```python
from build123d import *

# Parameters (mm, degrees)
SKETCH_1_R               = 9
SKETCH_1_R_2             = 6.25
EXTRUDE_1_DEPTH          = 200
SKETCH_2_R               = 1.75
CUT_EXTRUDE_1_DEPTH      = 10
CUT_EXTRUDE_1_DEPTH_BACK = 10


with BuildPart() as part:
    # ｽｹｯﾁ1 → ﾎﾞｽ - 押し出し1 (new body)
    with BuildSketch(Plane.XY):
        Circle(SKETCH_1_R)
        Circle(SKETCH_1_R_2, mode=Mode.SUBTRACT)
    extrude(amount=EXTRUDE_1_DEPTH)

    # ｽｹｯﾁ2 → ｶｯﾄ - 押し出し1 (cut, two sides)
    with BuildSketch(Plane(origin=(0, 0, 0), x_dir=(0, 0, -1), z_dir=(1, 0, 0))) as cut_extrude_1_sk:
        with Locations((-7.5, 0)):
            Circle(SKETCH_2_R)
        with Locations((-192.5, 0)):
            Circle(SKETCH_2_R)
    extrude(amount=CUT_EXTRUDE_1_DEPTH, mode=Mode.SUBTRACT)
    extrude(cut_extrude_1_sk.sketch, amount=-CUT_EXTRUDE_1_DEPTH_BACK, mode=Mode.SUBTRACT)


solid = part.part
```
Design review of the part built by this model. Coordinates are the model's own, in mm. Coordinates: 2 decimals unless noted, no trailing zeros. Write each loop counter-clockwise with the first axis right and the second up, starting at its lowest first coordinate (ties: lowest second). Pieces come first, ordered by that corner, then holes.
1) Add section A-A (y = 0). Write out the cut boundary in (x, z).
2) Add section B-B (z = 192.5). Write out the cut boundary in (x, y).
3) Mouldability with a two-part tool opening along Y and no side actions: class faces 1 (the cylindrical face through (7.479, 1.735, 192.728)), 2 (the cylindrical face through (-1.172, 8.923, 98.6)), 3 (the flat face through (-6.13, -1.87, 0)) as +Y half, -Y half, draft (parallel to the pull), parting line (faces both ways), or undercut.
4) Insertion check: pin 1 (3 mm diameter, centred on y = 0, z = 192.5, fed in from +X); pin 2 (1.5 mm diameter, centred on y = 2, z = 70, fed in from +X); pin 3 (2 mm diameter, centred on y = -6.5, z = 73.5, fed in from +X); pin 4 (1.5 mm diameter, centred on y = 3, z = 165.5, fed in from +X). Each pin has a flat end and moves straight along its axis. Give the tip position at first contact, or say it passes through.
5) To check wall thickness, follow L1, parallel to Y at x = 0, z = 52.5; L2, parallel to Z at x = 8, y = 0.75; L3, parallel to X at y = 6.5, z = 161.5. State the ranges of each line that lie inside material, in increasing order.
6) Add section D-D (z = 123). Write out the cut boundary in (x, y), plus the area to 3 significant figures.
7) Add section C-C (x = 2.5). Write out the cut boundary in (y, z).
Check result:
1. outline: (-9, 0) - (-6.25, 0) - (-6.25, 5.75) - (-9, 5.75) - close; (-9, 9.25) - (-6.25, 9.25) - (-6.25, 190.75) - (-9, 190.75) - close; (-9, 194.25) - (-6.25, 194.25) - (-6.25, 200) - (-9, 200) - close; (6.25, 0) - (9, 0) - (9, 5.75) - (6.25, 5.75) - close; (6.25, 9.25) - (9, 9.25) - (9, 190.75) - (6.25, 190.75) - close; (6.25, 194.25) - (9, 194.25) - (9, 200) - (6.25, 200) - close
2. outline: (-8.83, -1.75) arc R9 ccw to (8.83, -1.75) - (6, -1.75) arc R6.25 cw to (-6, -1.75) - close; (-8.83, 1.75) - (-6, 1.75) arc R6.25 cw to (6, 1.75) - (8.83, 1.75) arc R9 ccw to start
3. face 1: undercut
3. face 2: parting line
3. face 3: draft
4. pin 1: passes through
4. pin 2: stops at x = 8.91
4. pin 3: stops at x = 7.12
4. pin 4: stops at x = 8.71
5. L1: y = -9 to -6.25, 6.25 to 9
5. L2: z = 0 to 5.92, 9.08 to 190.92, 194.08 to 200
5. L3: x = -6.22 to 6.22
6. outline: circle Ø18 at (0, 0); hole circle Ø12.5 at (0, 0)
6. area: 132 mm2
7. outline: (-8.65, 0) - (-5.73, 0) - (-5.73, 200) - (-8.65, 200) - close; (5.73, 0) - (8.65, 0) - (8.65, 200) - (5.73, 200) - close
